from build123d import *

# Parameters (mm, degrees)
SKETCH_1_W           = 158.76721969
SKETCH_1_H           = 156
EXTRUDE_1_DEPTH      = 65
SKETCH_2_W           = 158.85328248
SKETCH_2_H           = 116
CUT_EXTRUDE_1_DEPTH  = 175.106359002
SKETCH_3_W           = 50.908374927
SKETCH_3_H           = 145.199783254
CUT_EXTRUDE_2_DEPTH  = 30
SKETCH_4_W           = 35
SKETCH_4_H           = 35
CUT_EXTRUDE_3_DEPTH  = 6
SKETCH_5_W           = 15
SKETCH_5_H           = 7
CUT_EXTRUDE_4_DEPTH  = 30
SKETCH_6_W           = 16.173646408
SKETCH_6_H           = 21.728169507
CUT_EXTRUDE_5_DEPTH  = 10
SKETCH_12_W          = 86.243953328
SKETCH_12_H          = 39.310546327
CUT_EXTRUDE_8_DEPTH  = 175.106359002
SKETCH_9_W           = 48
SKETCH_9_H           = 24
CUT_EXTRUDE_6_DEPTH  = 65
SKETCH_10_W          = 13
SKETCH_10_H          = 21.606977086
CUT_EXTRUDE_7_DEPTH  = 142
SKETCH_14_W          = 115.071710401
SKETCH_14_H          = 109.204529419
CUT_EXTRUDE_9_DEPTH  = 183.843220343
SKETCH_17_W          = 7.5
SKETCH_17_H          = 137.87
EXTRUDE_2_DEPTH      = 4
SKETCH_16_R          = 1.5
CUT_EXTRUDE_10_DEPTH = 182.230387146
SKETCH_18_W          = 105.560370757
SKETCH_18_H          = 69.761390661
CUT_EXTRUDE_11_DEPTH = 10
SKETCH_20_W          = 34.311797321
SKETCH_20_H          = 49.303612094
CUT_EXTRUDE_12_DEPTH = 20
SKETCH_21_R          = 1.5
CUT_EXTRUDE_13_DEPTH = 15
SKETCH_22_W          = 34.558218505
SKETCH_22_H          = 17.119534262
CUT_EXTRUDE_14_DEPTH = 15
SKETCH_23_R          = 1.5
CUT_EXTRUDE_15_DEPTH = 15
SKETCH_28_R          = 1.6
CUT_EXTRUDE_17_DEPTH = 10
FILLET_5_R           = 10
FILLET_6_R           = 10
SKETCH_24_R          = 42.345367042
SKETCH_24_R_2        = 32.5
EXTRUDE_3_DEPTH      = 15
EXTRUDE_START        = 15
EXTRUDE_4_DEPTH      = 15
EXTRUDE_5_DEPTH      = 15
SKETCH_31_W          = 132.972003353
SKETCH_31_H          = 50.361945542
CUT_EXTRUDE_18_DEPTH = 15


with BuildPart() as part:
    # 草图1 → 凸台-拉伸1 (new body)
    with BuildSketch(Plane(origin=(0, 0, 0), x_dir=(0, 0, -1), z_dir=(1, 0, 0))):
        with Locations((-21.604044476, 48.053631124)):
            Rectangle(SKETCH_1_W, SKETCH_1_H)
    extrude(amount=EXTRUDE_1_DEPTH)

    # 草图2 → 切除-拉伸1 (cut, through all)
    with BuildSketch(Plane(origin=(65, 0, 0), x_dir=(0, 0, -1), z_dir=(1, 0, 0))):
        with Locations((18.438986919, 28.053631124)):
            Rectangle(SKETCH_2_W, SKETCH_2_H)
    extrude(amount=-CUT_EXTRUDE_1_DEPTH, mode=Mode.SUBTRACT)

    # 草图3 → 切除-拉伸2 (cut)
    with BuildSketch(Plane.XY.offset(100.987654321)):
        with Locations((33.848978786, 39.12697696)):
            Rectangle(SKETCH_3_W, SKETCH_3_H)
    extrude(amount=-CUT_EXTRUDE_2_DEPTH, mode=Mode.SUBTRACT)

    # 草图4 → 切除-拉伸3 (cut)
    with BuildSketch(Plane(origin=(0, 126.053631124, 0), x_dir=(1, 0, 0), z_dir=(0, 1, 0))):
        with Locations((36.50386385, -33.487654321)):
            Rectangle(SKETCH_4_W, SKETCH_4_H)
    extrude(amount=-CUT_EXTRUDE_3_DEPTH, mode=Mode.SUBTRACT)

    # 草图5 → 切除-拉伸4 (cut)
    with BuildSketch(Plane(origin=(0, 120.053631124, 0), x_dir=(1, 0, 0), z_dir=(0, 1, 0))):
        with Locations((36.50386385, -47.487654321)):
            Rectangle(SKETCH_5_W, SKETCH_5_H)
    extrude(amount=-CUT_EXTRUDE_4_DEPTH, mode=Mode.SUBTRACT)

    # 草图6 → 切除-拉伸5 (cut)
    with BuildSketch(Plane.XY.offset(70.987654321)):
        with Locations((36.425330815, 100.862783834)):
            Rectangle(SKETCH_6_W, SKETCH_6_H)
    extrude(amount=-CUT_EXTRUDE_5_DEPTH, mode=Mode.SUBTRACT)

    # 草图12 → 切除-拉伸8 (cut, through all)
    with BuildSketch(Plane(origin=(65, 0, 0), x_dir=(0, 0, -1), z_dir=(1, 0, 0))):
        with Locations((-69.77461077, -31.47164204)):
            Rectangle(SKETCH_12_W, SKETCH_12_H)
    extrude(amount=-CUT_EXTRUDE_8_DEPTH, mode=Mode.SUBTRACT)

    # 草图9 → 切除-拉伸6 (cut)
    with BuildSketch(Plane(origin=(0, 0, -57.779565369), x_dir=(-1, 0, 0), z_dir=(0, 0, -1))):
        with Locations((-35.359469061, 106.501927087)):
            Rectangle(SKETCH_9_W, SKETCH_9_H)
    extrude(amount=-CUT_EXTRUDE_6_DEPTH, mode=Mode.SUBTRACT)

    # 草图10 → 切除-拉伸7 (cut)
    with BuildSketch(Plane(origin=(0, 0, 7.220434631), x_dir=(-1, 0, 0), z_dir=(0, 0, -1))):
        with Locations((-17.859469061, 105.30541563)):
            Rectangle(SKETCH_10_W, SKETCH_10_H)
    extrude(amount=-CUT_EXTRUDE_7_DEPTH, mode=Mode.SUBTRACT)

    # 草图14 → 切除-拉伸9 (cut, through all)
    with BuildSketch(Plane(origin=(0, 126.053631124, 0), x_dir=(1, 0, 0), z_dir=(0, 1, 0))):
        with Locations((38.012225103, 53.381830079)):
            Rectangle(SKETCH_14_W, SKETCH_14_H)
    extrude(amount=-CUT_EXTRUDE_9_DEPTH, mode=Mode.SUBTRACT)

    # 草图17 → 凸台-拉伸2 (add)
    with BuildSketch(Plane.XY.offset(100.987654321)):
        with Locations((-3.75, 57.118631124)):
            Rectangle(SKETCH_17_W, SKETCH_17_H)
        with Locations((68.75, 57.118631124)):
            Rectangle(SKETCH_17_W, SKETCH_17_H)
    extrude(amount=-EXTRUDE_2_DEPTH)

    # 草图16 → 切除-拉伸10 (cut, through all)
    with BuildSketch(Plane(origin=(0, 120.053631124, 0), x_dir=(1, 0, 0), z_dir=(0, 1, 0))):
        with Locations(Location((24.95386385, -46.987654321, 0), (0, 0, 270))):
            Circle(SKETCH_16_R)
        with Locations(Location((48.05386385, -46.987654321, 0), (0, 0, 270))):
            Circle(SKETCH_16_R)
        with Locations(Location((24.95386385, -23.987654321, 0), (0, 0, 270))):
            Circle(SKETCH_16_R)
        with Locations(Location((48.05386385, -23.987654321, 0), (0, 0, 270))):
            Circle(SKETCH_16_R)
    extrude(amount=-CUT_EXTRUDE_10_DEPTH, mode=Mode.SUBTRACT)

    # 草图18 → 切除-拉伸11 (cut)
    with BuildSketch(Plane.XZ.offset(-86.053631124)):
        with Locations((39.446315854, 26.113971664)):
            Rectangle(SKETCH_18_W, SKETCH_18_H)
    extrude(amount=-CUT_EXTRUDE_11_DEPTH, mode=Mode.SUBTRACT)

    # 草图20 → 切除-拉伸12 (cut)
    with BuildSketch(Plane.XZ.offset(-96.053631124)):
        with Locations((41.515367722, 36.342860947)):
            Rectangle(SKETCH_20_W, SKETCH_20_H)
    extrude(amount=-CUT_EXTRUDE_12_DEPTH, mode=Mode.SUBTRACT)

    # 草图21 → 切除-拉伸13 (cut)
    with BuildSketch(Plane(origin=(0, 0, 7.220434631), x_dir=(-1, 0, 0), z_dir=(0, 0, -1))):
        with Locations((-52.200258978, 114.424449587)):
            Circle(SKETCH_21_R)
        with Locations((-52.210974666, 99.924453546)):
            Circle(SKETCH_21_R)
    extrude(amount=-CUT_EXTRUDE_13_DEPTH, mode=Mode.SUBTRACT)

    # 草图22 → 切除-拉伸14 (cut)
    with BuildSketch(Plane.XY.offset(70.987654321)):
        with Locations((41.638578314, 103.167101456)):
            Rectangle(SKETCH_22_W, SKETCH_22_H)
    extrude(amount=-CUT_EXTRUDE_14_DEPTH, mode=Mode.SUBTRACT)

    # 草图23 → 切除-拉伸15 (cut)
    with BuildSketch(Plane.XY.offset(100.987654321)):
        with Locations((69, 116.053631124)):
            Circle(SKETCH_23_R)
        with Locations((69, 86.053631124)):
            Circle(SKETCH_23_R)
        with Locations((69, 46.053631124)):
            Circle(SKETCH_23_R)
        with Locations((69, 16.053631124)):
            Circle(SKETCH_23_R)
        with Locations((-4, 116.053631124)):
            Circle(SKETCH_23_R)
        with Locations((-4, 86.053631124)):
            Circle(SKETCH_23_R)
        with Locations((-4, 46.053631124)):
            Circle(SKETCH_23_R)
        with Locations((-4, 16.053631124)):
            Circle(SKETCH_23_R)
    extrude(amount=-CUT_EXTRUDE_15_DEPTH, mode=Mode.SUBTRACT)

    # 草图28 → 切除-拉伸17 (cut)
    with BuildSketch(Plane.XY.offset(70.987654321)):
        with Locations((16.622657387, 69.823755444)):
            Circle(SKETCH_28_R)
        with Locations((52.182657387, 69.823755444)):
            Circle(SKETCH_28_R)
        with Locations((16.622657387, 44.803755444)):
            Circle(SKETCH_28_R)
        with Locations((52.182657387, 44.803755444)):
            Circle(SKETCH_28_R)
    extrude(amount=-CUT_EXTRUDE_17_DEPTH, mode=Mode.SUBTRACT)

    # 圆角5
    fillet_5_edges = [part.edges().sort_by_distance(p)[0] for p in [
        (0, 126.053631124, 49.104044476),
        (65, 126.053631124, 49.104044476),
    ]]
    fillet(fillet_5_edges, radius=FILLET_5_R)

    # 圆角6
    # the kernel refuses this fillet: 10 mm, written as the material it takes off along each edge
    with BuildSketch(Plane(origin=(65, 96.053631124, 60.994666994), x_dir=(-1, 0, 0), z_dir=(0, 0, -1)), Plane(origin=(0, 96.053631124, 60.994666994), x_dir=(0, 1, 0), z_dir=(0, 0, -1))) as fillet_6_piece_1:
        with BuildLine():
            CenterArc((FILLET_6_R, FILLET_6_R), FILLET_6_R, 180, 90)
            Line((0, FILLET_6_R), (0, 0))
            Line((0, 0), (FILLET_6_R, 0))
        make_face()
    extrude(amount=84.774232362, mode=Mode.SUBTRACT)

    # 草图24 → 凸台-拉伸3 (add)
    with BuildSketch(Plane.XZ.offset(11.816368876)):
        with Locations(Location((32.330540247, 100.987654321, 0), (0, 0, 320.488798593))):
            Circle(SKETCH_24_R)
        with Locations((32.330540247, 100.987654321)):
            Circle(SKETCH_24_R_2, mode=Mode.SUBTRACT)
    extrude(amount=EXTRUDE_3_DEPTH)

    # 草图29 → 凸台-拉伸4 (add)
    with BuildSketch(Plane(origin=(0, -11.816368876, 0), x_dir=(1, 0, 0), z_dir=(0, 1, 0)).offset(EXTRUDE_START)):
        with BuildLine():
            Line((0, -73.640510462), (0, -96.784474951))
            Line((0, -96.784474951), (-9.805707724, -96.784474951))
            ThreePointArc((-9.805707724, -96.784474951), (-6.659668908, -84.468159778), (0, -73.640510462))
        make_face()
    extrude(amount=-EXTRUDE_4_DEPTH)

    # 草图30 → 凸台-拉伸5 (add)
    with BuildSketch(Plane(origin=(0, -11.816368876, 0), x_dir=(1, 0, 0), z_dir=(0, 1, 0)).offset(EXTRUDE_START)):
        with BuildLine():
            Line((74.449305819, -96.612760422), (65, -96.987654321))
            Line((65, -96.987654321), (65, -74.046301175))
            ThreePointArc((65, -74.046301175), (71.389866055, -84.632252236), (74.449305819, -96.612760422))
        make_face()
    extrude(amount=-EXTRUDE_5_DEPTH)

    # 草图31 → 切除-拉伸18 (cut)
    with BuildSketch(Plane(origin=(0, -11.816368876, 0), x_dir=(1, 0, 0), z_dir=(0, 1, 0))):
        with Locations((46.807884266, -126.3437758)):
            Rectangle(SKETCH_31_W, SKETCH_31_H)
    extrude(amount=-CUT_EXTRUDE_18_DEPTH, mode=Mode.SUBTRACT)


solid = part.part
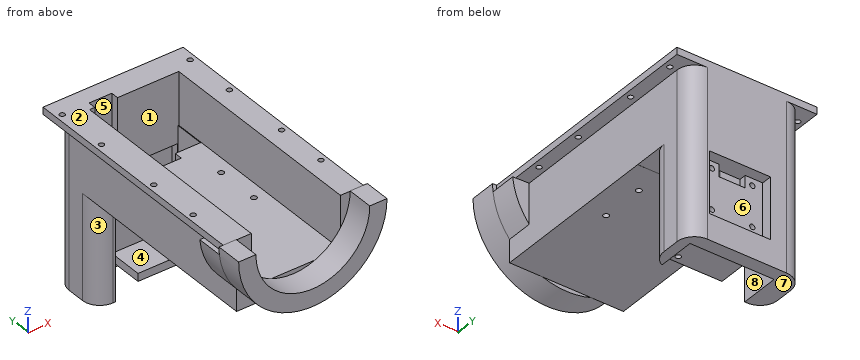
Input: part model. Units: mm. Frame: model coordinates. Face numbers are marked on the shaded views. A direction names the side the tool comes from. Coordinates: 2 decimals unless noted, no trailing zeros. Loops run counter-clockwise (first coordinate to the right, second up) from the corner with the lowest first, then second, coordinate; pieces in that order, holes last.
Q1. Cut plane D-D (y = -7). Output: boundary loops of the cut face in (x, z).
Q2. Cut plane A-A (y = 109). Output: boundary loops of the cut face in (x, z).
Q3. Set-up query: the marked faces 1, 2, 3, 4 and 5. Return all of +Z, -Z, +X, -X, +Y, -Y with unobstructed straight access to the full face (end or side cutting, diameter ignored); none if empty.
Q4. Cut plane C-C (x = 33). Give the number of separate pieces and of enclosed holes in the cut face, then the cut area to 3 significant figures.
Q5. Cut plane B-B (z = 54). Output: boundary loops of the cut face in (x, y), then the cut area to 3 significant figures.
Q6. Material intervals for line 1 (Y direction, x = 69, z = 98.6); line 2 (X direction, y = 6.5, z = 74); line 3 (X direction, y = 96, z = 69), sorted ascending.
Q7. Contact query for flat-ended pins moving along their axis: pin 1 (1 mm diameter, centred on y = 56.5, z = 79.5, fed in from -X); pin 2 (1.8 mm diameter, centred on y = 123, z = 26, fed in from -X) (3 decimals); pin 3 (7 mm diameter, centred on y = 105, z = 36.5, fed in from +X); pin 4 (1.8 mm diameter, centred on x = 69, y = 86.05, fed in from -Z). Output: stop coordinate, or through.
Q8. Draft query along Z for the marked faces 6, 7 and 8. Return one class per face: +Z half, -Z half, draft (parallel to the pull), parting line (faces both ways), or undercut.
Working result:
1. outline: (-9.81, 96.78) arc R42.35 ccw to (0, 73.64) - (0, 60.99) - (65, 60.99) - (65, 74.05) arc R42.35 ccw to (74.45, 96.61) - (65, 96.99) - (72.5, 96.99) - (72.5, 100.99) - (59.3, 100.99) - (59.3, 70.99) - (8.39, 70.99) - (8.39, 100.99) - (-7.5, 100.99) - (-7.5, 96.99) - (0, 96.99) - (0, 96.78) - close
2. outline: (-7.5, 96.99) - (0, 96.99) - (0, 1.22) - (11.36, 1.22) - (11.36, 70.99) - (8.39, 70.99) - (8.39, 100.99) - (-7.5, 100.99) - close; (24.36, 7.22) - (59.36, 7.22) - (59.36, 1.22) - (65, 1.22) - (65, 96.99) - (72.5, 96.99) - (72.5, 100.99) - (59.3, 100.99) - (59.3, 70.99) - (58.92, 70.99) - (58.92, 55.99) - (58.67, 55.99) - (58.67, 11.69) - (24.36, 11.69) - close
3. face 1: +Z
3. face 2: +Z, +X, -X, +Y
3. face 3: -Z, -X, -Y
3. face 4: -Y
3. face 5: +Z, -Z
4. separate pieces: 3
4. enclosed holes: 0
4. area: 2,170 mm2
5. outline: (0, 106.05) arc R10 ccw to (10, 96.05) - (11.36, 96.05) - (11.36, 116.11) - (24.36, 116.11) - (24.36, 116.05) - (58.67, 116.05) - (58.67, 96.75) arc R10 ccw to (65, 106.05) - (65, 116.05) arc R10 ccw to (55, 126.05) - (10, 126.05) arc R10 ccw to (0, 116.05) - close
5. area: 918 mm2
6. line 1: y = -26.82 to 14.55, 17.55 to 44.55, 47.55 to 84.55, 87.55 to 114.55, 117.55 to 126.05
6. line 2: x = 0 to 8.39, 59.3 to 65
6. line 3: x = 0 to 11.36, 58.92 to 65
7. pin 1: stops at x = 0
7. pin 2: stops at x = 2.035
7. pin 3: stops at x = 65
7. pin 4: passes through
8. face 6: undercut
8. face 7: -Z half
8. face 8: draft
